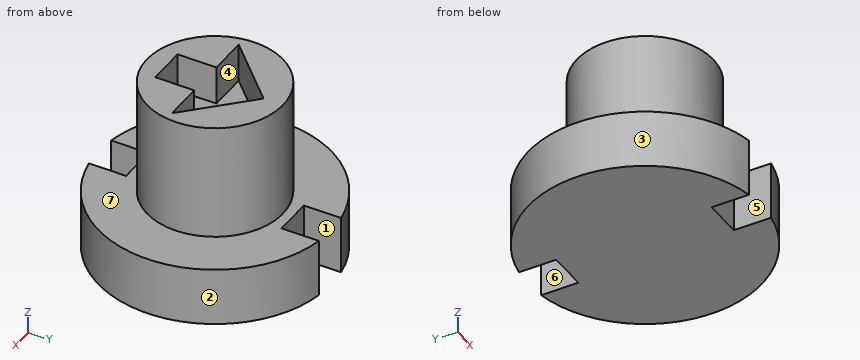
```python
from build123d import *

# Parameters (mm, degrees)
CROQUIS1_R              = 3.5
SALIENTE_EXTRUIR1_DEPTH = 6
CROQUIS2_R              = 6
SALIENTE_EXTRUIR2_DEPTH = 3
CORTAR_EXTRUIR1_DEPTH   = 2
CROQUIS4_W              = 2
CROQUIS4_H              = 2
CORTAR_EXTRUIR2_DEPTH   = 4


with BuildPart() as part:
    # Croquis1 → Saliente-Extruir1 (new body)
    with BuildSketch(Plane.XY):
        with Locations((-4.754102012, 3.97833761)):
            Circle(CROQUIS1_R)
    extrude(amount=SALIENTE_EXTRUIR1_DEPTH)

    # Croquis2 → Saliente-Extruir2 (add)
    with BuildSketch(Plane(origin=(0, 0, 0), x_dir=(-1, 0, 0), z_dir=(0, 0, -1))):
        with Locations((4.754102012, 3.97833761)):
            Circle(CROQUIS2_R)
    extrude(amount=SALIENTE_EXTRUIR2_DEPTH)

    # Croquis3 → Cortar-Extruir1 (cut)
    with BuildSketch(Plane.XY.offset(6)):
        Polygon((-5.754102012, 1.47833761), (-3.754102012, 1.47833761), (-3.754102012, 3.47833761), (-1.754102012, 3.47833761), (-4.754102012, 6.47833761), (-7.754102012, 3.47833761), (-5.754102012, 3.47833761), align=None)
    extrude(amount=-CORTAR_EXTRUIR1_DEPTH, mode=Mode.SUBTRACT)

    # Croquis4 → Cortar-Extruir2 (cut, through all)
    with BuildSketch(Plane.XY):
        with Locations((-4.754102012, 8.97833761)):
            Rectangle(CROQUIS4_W, CROQUIS4_H)
        Polygon((-5.754102012, -0.02166239), (-3.754102012, -0.02166239), (-3.754102012, -2.02166239), (-4.754102012, -2.02166239), (-5.754102012, -2.02166239), align=None)
    extrude(amount=-CORTAR_EXTRUIR2_DEPTH, mode=Mode.SUBTRACT)


solid = part.part
```
Geometry check sheet. Reference: the model listing, model coordinates, mm. Face numbers are marked on the shaded views. A direction names the side the tool comes from. Round coordinates to 2 decimals unless told otherwise and drop trailing zeros. Write each loop counter-clockwise with the first axis right and the second up, starting at its lowest first coordinate (ties: lowest second). Pieces come first, ordered by that corner, then holes. Notation, with made-up numbers: (73.25, -19.75) -> (103.25, -19.75) arc R13 cw to (103.25, -11.75) -> close; hole circle Ø9 at (-18.75, 30). An arc over 180 degrees is marked (long way). Put each result on its own line as item: value.
1) Depth check by flat-ended pin: P1, Ø1.5, axis at y = 8.5, z = -1.5, coming from the +X side; P2, Ø1, axis at y = 2, z = 5, coming from the +X side; P3, Ø0.6, axis at x = -6.5, z = 5, coming from the +Y side. Enter the tip coordinate at first touch or a pass-through.
Recorded:
P1: stops at x = -0.09
P2: stops at x = -1.58
P3: stops at y = 7.17
2) Cross-section at D-D, the plane y = 8.25. Enter the section's corners in (x, z), plus the area to 3 significant figures.
Recorded:
outline: (-8.97, -3) -> (-5.75, -3) -> (-5.75, 0) -> (-8.97, 0) -> close; (-3.75, -3) -> (-0.54, -3) -> (-0.54, 0) -> (-3.75, 0) -> close
area: 19.3 mm2
3) Release check for a two-part mould opening along X. For the marked faces 1, 2, 3 and 4 record: pulls with the +X half, pulls with the -X half, needs draft (parallel to the pull), parting line crosses it, or undercut.
Recorded:
face 1: undercut
face 2: pulls with the +X half
face 3: pulls with the -X half
face 4: undercut
4) Access from +Z, -Z, +X, -X, +Y, -Y to the whole of each face (thin tool, end or side, straight path). Record for the marked faces 5, 6 and 7.
Recorded:
face 5: +Z, -Z, -Y
face 6: +Z, -Z, +Y
face 7: +Z
5) Cross-section at C-C, the plane x = -5.5. Enter the section's corners in (y, z).
Recorded:
outline: (-0.02, -3) -> (7.98, -3) -> (7.98, 0) -> (7.4, 0) -> (7.4, 6) -> (5.73, 6) -> (5.73, 4) -> (1.48, 4) -> (1.48, 6) -> (0.56, 6) -> (0.56, 0) -> (-0.02, 0) -> close
6) Cross-section at B-B, the plane y = 5. Enter the section's corners in (x, z), plus the area to 3 significant figures.
Recorded:
outline: (-10.67, -3) -> (1.16, -3) -> (1.16, 0) -> (-1.41, 0) -> (-1.41, 6) -> (-3.28, 6) -> (-3.28, 4) -> (-6.23, 4) -> (-6.23, 6) -> (-8.1, 6) -> (-8.1, 0) -> (-10.67, 0) -> close
area: 69.7 mm2
7) Thickness scan on probe 1 along Z at (x, y) = (-5, 2.5); probe 2 along Z at (x, y) = (-3.25, 0.25); probe 3 along X at (y, z) = (8.5, -1.5). Record the ranges inside material, lowest first. Write a range as from..to.
Recorded:
probe 1: z = -3..4
probe 2: z = -3..0
probe 3: x = -8.7..-5.75, -3.75..-0.81
8) Cross-section at A-A, the plane z = -2. Enter the section's corners in (x, y).
Recorded:
outline: (-5.75, -1.94) -> (-5.75, -0.02) -> (-3.75, -0.02) -> (-3.75, -1.94) arc R6 ccw to (-3.75, 9.89) -> (-3.75, 7.98) -> (-5.75, 7.98) -> (-5.75, 9.89) arc R6 ccw to start
